```python
from build123d import *

# Parameters (mm, degrees)
SKETCH1_R           = 50.8
BOSS_EXTRUDE1_DEPTH = 889
EXTRUDE_THIN1_DEPTH = 101.6
FILLET1_R           = 2.54


with BuildPart() as part:
    # Sketch1 → Boss-Extrude1 (new body)
    with BuildSketch(Plane.XY):
        Circle(SKETCH1_R)
    extrude(amount=-BOSS_EXTRUDE1_DEPTH)

    # Sketch3 → Extrude-Thin1 (add, symmetric)
    with BuildSketch(Plane(origin=(0, 0, 0), x_dir=(1, 0, 0), z_dir=(0, 1, 0))):
        Polygon((254, 0), (-254, 0), (-254, 635), (-279.4, 635), (-279.4, -25.4), (254, -25.4), align=None)
    extrude(amount=EXTRUDE_THIN1_DEPTH, both=True)

    # Fillet1
    fillet1_edges = [part.edges().sort_by_distance(p)[0] for p in [
        (-50.8, 0, 0),
        (-50.8, 0, -889),
        (-254, -101.6, -317.5),
        (-254, 0, 0),
        (-254, 0, -635),
        (-279.4, 101.6, -304.8),
        (-279.4, 0, -635),
        (-12.7, 101.6, 25.4),
        (-279.4, 0, 25.4),
        (254, 0, 25.4),
        (0, -101.6, 0),
        (254, 0, 0),
        (-254, 101.6, -317.5),
        (0, 101.6, 0),
        (-12.7, -101.6, 25.4),
        (-279.4, -101.6, -304.8),
    ]]
    fillet(fillet1_edges, radius=FILLET1_R)


solid = part.part
```
Model file for the job. Use its own axes, mm. A direction names the side the tool comes from. Coordinates: 2 decimals unless noted, no trailing zeros. Write each loop counter-clockwise with the first axis right and the second up, starting at its lowest first coordinate (ties: lowest second). Pieces come first, ordered by that corner, then holes. Notation, with made-up numbers: (5, 57.5) - (43, 57.5) arc R19 ccw to (43, 78.5) - close; hole circle Ø3 at (8, -1). An arc over 180 degrees is marked (long way). One line per question, with ' | ' between items. Start each with the question number.
Q1. Cut at D-D, the plane x = 0. List the corners of the cut face in (y, z), then the cut area to 3 significant figures.
Q2. Pin check, flat tips, straight feed: pin 1 (12 mm diameter, centred on y = 23.5, z = -665, fed in from -X); pin 2 (2 mm diameter, centred on y = -57.5, z = -314, fed in from +X); pin 3 (6 mm diameter, centred on x = -267, y = 32.5, fed in from -Z). Stop position of each tip, or through.
Q3. Cut at B-B, the plane x = 122. List the corners of the cut face in (y, z), then the cut area to 3 significant figures.
Q4. Cut at C-C, the plane y = 0. List the corners of the cut face in (x, z), then the cut area to 3 significant figures.
Q5. Pull direction X, two halves, no side cores. Call faces 1 (the face through (-11.012, -49.592, -438.313)), 2 (the face through (-268, 101.6, -161)), 3 (the face through (254, 1, 13)): pulls with the +X half, pulls with the -X half, needs draft (parallel to the pull), parting line crosses it, or undercut.
Q6. Cut at A-A, the plane z = -317. List the corners of the cut face in (x, y).
Q7. Drill centre lines: line 1 (Y direction, x = 1, z = -793); line 2 (Z direction, x = 43, y = -75); line 3 (X direction, y = 56.5, z = -126.5). Where is each one in solid material? Low to high. Write a range as [from, to].
Q8. 3-axis set-ups, long thin cutter, end or side, ignore diameter. For faces 4 (the face through (-279.4, 1, -309)), 5 (the face through (-254, 1, -313)), 6 (the face through (-267, 1, -635)): which of +Z, -Z, +X, -X, +Y, -Y reach the whole face in a straight line?
Answer below:
1) outline: (-101.6, 2.54) arc R2.54 ccw to (-99.06, 0) - (-53.34, 0) arc R2.54 cw to (-50.8, -2.54) - (-50.8, -886.46) arc R2.54 ccw to (-48.26, -889) - (48.26, -889) arc R2.54 ccw to (50.8, -886.46) - (50.8, -2.54) arc R2.54 cw to (53.34, 0) - (99.06, 0) arc R2.54 ccw to (101.6, 2.54) - (101.6, 22.86) arc R2.54 ccw to (99.06, 25.4) - (-99.06, 25.4) arc R2.54 ccw to (-101.6, 22.86) - close | area: 95,500 mm^2
2) pin 1: x = -47.69 | pin 2: x = -254 | pin 3: z = -635
3) outline: (-101.6, 2.54) arc R2.54 ccw to (-99.06, 0) - (99.06, 0) arc R2.54 ccw to (101.6, 2.54) - (101.6, 22.86) arc R2.54 ccw to (99.06, 25.4) - (-99.06, 25.4) arc R2.54 ccw to (-101.6, 22.86) - close | area: 5,160 mm^2
4) outline: (-279.4, -632.46) arc R2.54 ccw to (-276.86, -635) - (-256.54, -635) arc R2.54 ccw to (-254, -632.46) - (-254, -2.54) arc R2.54 cw to (-251.46, 0) - (-53.34, 0) arc R2.54 cw to (-50.8, -2.54) - (-50.8, -886.46) arc R2.54 ccw to (-48.26, -889) - (48.26, -889) arc R2.54 ccw to (50.8, -886.46) - (50.8, -2.54) arc R2.54 cw to (53.34, 0) - (251.46, 0) arc R2.54 ccw to (254, 2.54) - (254, 22.86) arc R2.54 ccw to (251.46, 25.4) - (-276.86, 25.4) arc R2.54 ccw to (-279.4, 22.86) - close | area: 120,000 mm^2
5) face 1: undercut | face 2: needs draft | face 3: pulls with the +X half
6) outline: (-279.4, -99.06) arc R2.54 ccw to (-276.86, -101.6) - (-256.54, -101.6) arc R2.54 ccw to (-254, -99.06) - (-254, 99.06) arc R2.54 ccw to (-256.54, 101.6) - (-276.86, 101.6) arc R2.54 ccw to (-279.4, 99.06) - close; circle Ø101.6 at (0, 0)
7) line 1: [-50.79, 50.79] | line 2: [0, 25.4] | line 3: [-279.4, -254]
8) face 4: +Z, -Z, -X, +Y, -Y | face 5: -Z, +Y, -Y | face 6: -Z, -X, +Y, -Y
